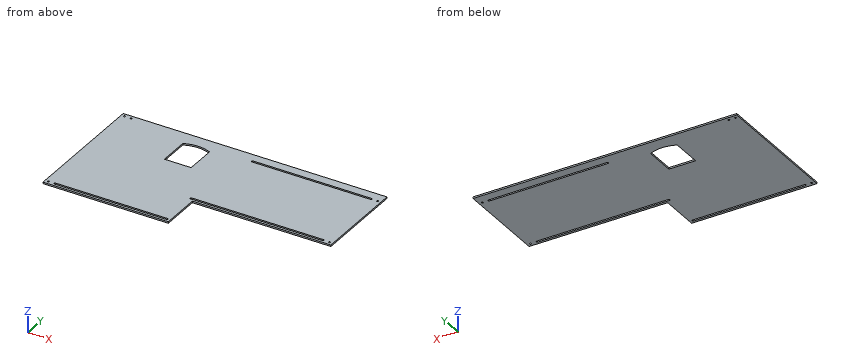
```python
from build123d import *

# Parameters (mm, degrees)
SKETCH_R      = 3.556
EXTRUDE_DEPTH = 5.9944


with BuildPart() as part:
    # Sketch → Extrude (new body)
    with BuildSketch(Plane.XY):
        Polygon((0, -508), (482.6, -508), (482.6, -355.6), (1016, -355.6), (1016, 0), (0, 0), align=None)
        with Locations((12.7, -12.7)):
            Circle(SKETCH_R, mode=Mode.SUBTRACT)
        with Locations((38.1, -12.7)):
            Circle(SKETCH_R, mode=Mode.SUBTRACT)
        with Locations((1003.3, -38.1)):
            Circle(SKETCH_R, mode=Mode.SUBTRACT)
        with Locations((1003.3, -342.9)):
            Circle(SKETCH_R, mode=Mode.SUBTRACT)
        with Locations((12.7, -495.3)):
            Circle(SKETCH_R, mode=Mode.SUBTRACT)
        with BuildLine():
            Line((266.065, -176.53), (368.935, -176.53))
            Line((368.935, -176.53), (368.935, -60.148744))
            ThreePointArc((368.935, -60.148744), (317.5, -48.768), (266.065, -60.148744))
            Line((266.065, -176.53), (266.065, -60.148744))
        make_face(mode=Mode.SUBTRACT)
        with BuildLine():
            Line((469.9, -346.456), (977.9, -346.456))
            ThreePointArc((977.9, -346.456), (981.456, -342.9), (977.9, -339.344))
            Line((469.9, -339.344), (977.9, -339.344))
            ThreePointArc((469.9, -339.344), (466.344, -342.9), (469.9, -346.456))
        make_face(mode=Mode.SUBTRACT)
        with BuildLine():
            Line((520.7, -34.544), (977.9, -34.544))
            ThreePointArc((977.9, -41.656), (981.456, -38.1), (977.9, -34.544))
            Line((520.7, -41.656), (977.9, -41.656))
            ThreePointArc((520.7, -34.544), (517.144, -38.1), (520.7, -41.656))
        make_face(mode=Mode.SUBTRACT)
        with BuildLine():
            Line((38.1, -491.744), (469.9, -491.744))
            ThreePointArc((469.9, -498.856), (473.456, -495.3), (469.9, -491.744))
            Line((38.1, -498.856), (469.9, -498.856))
            ThreePointArc((38.1, -491.744), (34.544, -495.3), (38.1, -498.856))
        make_face(mode=Mode.SUBTRACT)
    extrude(amount=EXTRUDE_DEPTH)


solid = part.part
```
Geometry: final body of the model. Coordinates: model frame, mm. Round coordinates to 2 decimals unless told otherwise and drop trailing zeros. Loops run counter-clockwise (first coordinate to the right, second up) from the corner with the lowest first, then second, coordinate; pieces in that order, holes last. Notation, with made-up numbers: (6, 73) -> (14, 73) arc R16 ccw to (14, 104) -> close; hole circle Ø1 at (48, 54). An arc over 180 degrees is marked (long way). Use one line per item in the form item = value. Start each with the question number.
1) Line query: L1, parallel to Y at x = 900, z = 0.9; L2, parallel to Y at x = 12.7, z = 1.35; L3, parallel to X at y = -495.3, z = 4.15. Output: solid intervals per line, ascending.
2) Section C-C on x = 777.5. Output: boundary loops of the cut face in (y, z), then the cut area to 3 significant figures.
3) Section A-A on y = -156.5. Output: boundary loops of the cut face in (x, z) (3 decimals), then the cut area to 3 significant figures.
4) Section D-D on y = -430. Output: boundary loops of the cut face in (x, z), then the cut area to 3 significant figures.
5) First-contact query: P1, Ø1.8, axis at x = 669.5, z = 4, coming from the -Y side; P2, Ø3, axis at x = 733.5, z = 4, coming from the +Y side. Flat tips, straight axial feed; report the tip coordinate or a pass-through.
6) Section B-B on z = 3.4. Give the number of separate pieces and of enclosed holes in the cut face, then the cut area to 3 significant figures.
Response:
q1.L1 = -355.6 to -346.46, -339.34 to -41.66, -34.54 to 0
q1.L2 = -508 to -498.86, -491.74 to -16.26, -9.14 to 0
q1.L3 = 0 to 9.14, 16.26 to 34.54, 473.46 to 482.6
q2.outline = (-355.6, 0) -> (-346.46, 0) -> (-346.46, 5.99) -> (-355.6, 5.99) -> close; (-339.34, 0) -> (-41.66, 0) -> (-41.66, 5.99) -> (-339.34, 5.99) -> close; (-34.54, 0) -> (0, 0) -> (0, 5.99) -> (-34.54, 5.99) -> close
q2.area = 2,050 mm^2
q3.outline = (0, 0) -> (266.065, 0) -> (266.065, 5.994) -> (0, 5.994) -> close; (368.935, 0) -> (1016, 0) -> (1016, 5.994) -> (368.935, 5.994) -> close
q3.area = 5,470 mm^2
q4.outline = (0, 0) -> (482.6, 0) -> (482.6, 5.99) -> (0, 5.99) -> close
q4.area = 2,890 mm^2
q5.P1 = -355.6
q5.P2 = 0
q6.separate_pieces = 1
q6.enclosed_holes = 9
q6.area = 412,000 mm^2
